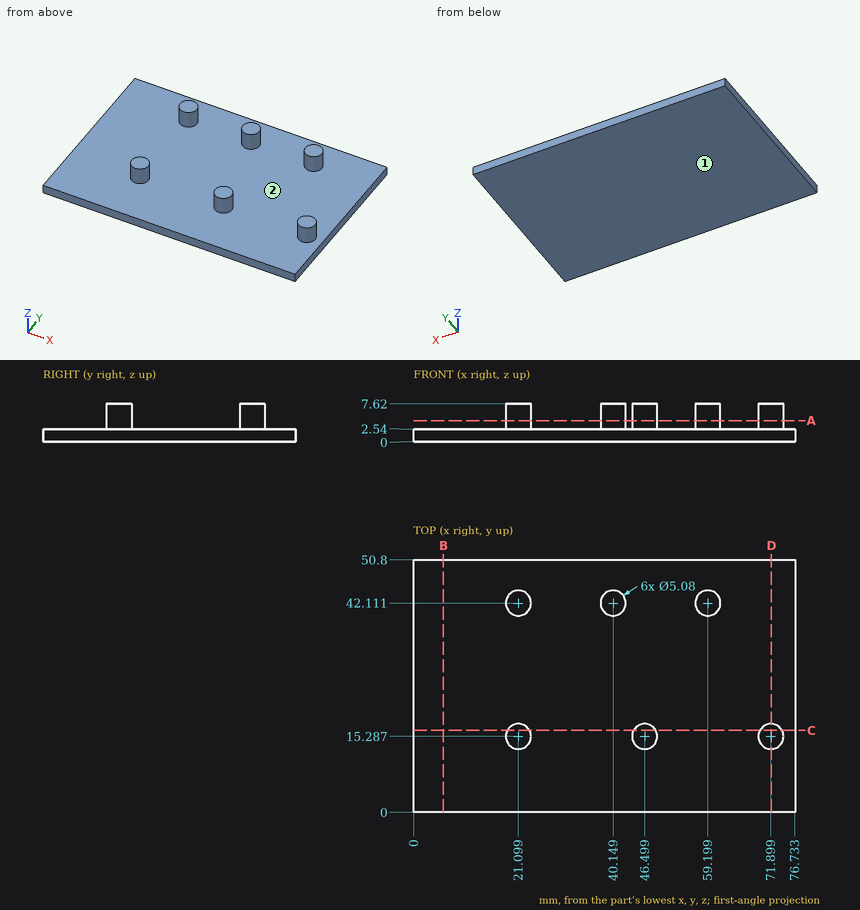
Design review of the part shown in the three views and the two pictorial views. Dimensions are in mm from the part's minimum x, y and z. Round coordinates to 2 decimals unless told otherwise and drop trailing zeros. Write each loop counter-clockwise with the first axis right and the second up, starting at its lowest first coordinate (ties: lowest second). Pieces come first, ordered by that corner, then holes.
Item 1: Draft analysis for pull direction Z (two halves, no side actions). For the marked faces 1 and 2, state which applies: released by +Z, released by -Z, zero draft, split by the parting line, or undercut.
Item 2: Consider section C-C on y = 16.5. Give the boundary of the cut face in (x, z).
Item 3: Consider section B-B on x = 6. Give the boundary of the cut face in (y, z).
Item 4: Consider section A-A on z = 4.25. Give the boundary of the cut face in (x, y), and give its area (3 significant figures).
Item 5: Wall thickness on L1, parallel to X at y = 15, z = 5 (1 decimal); L2, parallel to X at y = 41.5, z = 3.5 (1 decimal); L3, parallel to Z at x = 43.5, y = 20.5: over which ranges is each line inside the solid? List them lowest first.
Item 6: Consider section D-D on x = 72. Give the boundary of the cut face in (y, z) (1 decimal), and give its area (3 significant figures).
Check values:
1. face 1: released by -Z
1. face 2: released by +Z
2. outline: (0, 0) - (76.73, 0) - (76.73, 2.54) - (74.13, 2.54) - (74.13, 7.62) - (69.67, 7.62) - (69.67, 2.54) - (48.73, 2.54) - (48.73, 7.62) - (44.27, 7.62) - (44.27, 2.54) - (23.33, 2.54) - (23.33, 7.62) - (18.87, 7.62) - (18.87, 2.54) - (0, 2.54) - close
3. outline: (0, 0) - (50.8, 0) - (50.8, 2.54) - (0, 2.54) - close
4. outline: circle Ø5.08 at (21.1, 15.29); circle Ø5.08 at (21.1, 42.11); circle Ø5.08 at (40.15, 42.11); circle Ø5.08 at (46.5, 15.29); circle Ø5.08 at (59.2, 42.11); circle Ø5.08 at (71.9, 15.29)
4. area: 122 mm2
5. L1: x = 18.6 to 23.6, 44 to 49, 69.4 to 74.4
5. L2: x = 18.6 to 23.6, 37.7 to 42.6, 56.7 to 61.7
5. L3: z = 0 to 2.54
6. outline: (0, 0) - (50.8, 0) - (50.8, 2.5) - (17.8, 2.5) - (17.8, 7.6) - (12.7, 7.6) - (12.7, 2.5) - (0, 2.5) - close
6. area: 155 mm2
